Here's how the part is built. I have some questions about the finished solid (model axes, mm). A direction names the side the tool comes from. Give positions to 0.01 mm unless a question says otherwise; leave off trailing zeros. Loops run counter-clockwise (first coordinate to the right, second up) from the corner with the lowest first, then second, coordinate; pieces in that order, holes last. Notation, with made-up numbers: (43.25, 23) - (61.25, 23) arc R15 cw to (61.25, 51) - close; hole circle Ø2 at (-15.75, 38.25). An arc over 180 degrees is marked (long way). Use one line per item in the form item = value.
from build123d import *
from build123d.topology import SkipClean

# Parameters (mm, degrees)
ESBO_O1_R                = 11.15
RESSALTO_EXTRUS_O1_DEPTH = 15
ESBO_O2_R                = 22.5
RESSALTO_EXTRUS_O2_DEPTH = 4
RESSALTO_EXTRUS_O6_START = -8
ESBO_O5_R                = 11.15
ESBO_O5_R_2              = 8
RESSALTO_EXTRUS_O6_DEPTH = 8
RESSALTO_EXTRUS_O7_START = 4
ESBO_O7_R                = 14.2
ESBO_O7_R_2              = 11.15
RESSALTO_EXTRUS_O7_DEPTH = 4
RESSALTO_EXTRUS_O8_START = 4
ESBO_O8_R                = 11.15
ESBO_O8_R_2              = 8
RESSALTO_EXTRUS_O8_DEPTH = 4
RESSALTO_EXTRUS_O9_DEPTH = 7


with BuildPart() as part:
    # Esbo_o1 → Ressalto-extrus_o1 (new body)
    with BuildSketch(Plane.XY):
        with BuildLine():
            Line((-2.5, 18), (-2.5, 13.978197309))
            ThreePointArc((-2.5, 13.978197309), (-10.040916293, 10.040916293), (-13.978197309, 2.5))
            Line((-13.978197309, 2.5), (-18, 2.5))
            Line((-18, 2.5), (-18, -2.5))
            Line((-18, -2.5), (-13.978197309, -2.5))
            ThreePointArc((-13.978197309, -2.5), (-10.040916293, -10.040916293), (-2.5, -13.978197309))
            Line((-2.5, -13.978197309), (-2.5, -18))
            Line((-2.5, -18), (2.5, -18))
            Line((2.5, -18), (2.5, -13.978197309))
            ThreePointArc((2.5, -13.978197309), (10.040916293, -10.040916293), (13.978197309, -2.5))
            Line((13.978197309, -2.5), (18, -2.5))
            Line((18, -2.5), (18, 2.5))
            Line((18, 2.5), (13.978197309, 2.5))
            ThreePointArc((13.978197309, 2.5), (10.040916293, 10.040916293), (2.5, 13.978197309))
            Line((2.5, 13.978197309), (2.5, 18))
            Line((2.5, 18), (-2.5, 18))
        make_face()
        Circle(ESBO_O1_R, mode=Mode.SUBTRACT)
    extrude(amount=RESSALTO_EXTRUS_O1_DEPTH)

    # Esbo_o5 → Ressalto-extrus_o6 (add)
    with BuildSketch(Plane.XY.offset(15).offset(RESSALTO_EXTRUS_O6_START)):
        Circle(ESBO_O5_R)
        Circle(ESBO_O5_R_2, mode=Mode.SUBTRACT)
    extrude(amount=RESSALTO_EXTRUS_O6_DEPTH)



with BuildPart() as body_2:
    # Esbo_o2 → Ressalto-extrus_o2 (new body)
    # profile 1 of 5: a face of its own
    with SkipClean():  # the faces are left unmerged after this step: merging them gives an invalid solid
        with BuildSketch(Plane(origin=(0, 0, 0), x_dir=(-1, 0, 0), z_dir=(0, 0, -1))):
            Circle(ESBO_O2_R)
            with BuildLine():
                Line((2.5, 13.978197309), (2.5, 18))
                Line((2.5, 18), (-2.5, 18))
                Line((-2.5, 18), (-2.5, 13.978197309))
                ThreePointArc((-2.5, 13.978197309), (-10.040916293, 10.040916293), (-13.978197309, 2.5))
                Line((-13.978197309, 2.5), (-18, 2.5))
                Line((-18, 2.5), (-18, -2.5))
                Line((-18, -2.5), (-13.978197309, -2.5))
                ThreePointArc((-13.978197309, -2.5), (-10.040916293, -10.040916293), (-2.5, -13.978197309))
                Line((-2.5, -13.978197309), (-2.5, -18))
                Line((-2.5, -18), (2.5, -18))
                Line((2.5, -18), (2.5, -13.978197309))
                ThreePointArc((2.5, -13.978197309), (10.040916293, -10.040916293), (13.978197309, -2.5))
                Line((13.978197309, -2.5), (18, -2.5))
                Line((18, -2.5), (18, 2.5))
                Line((18, 2.5), (13.978197309, 2.5))
                ThreePointArc((13.978197309, 2.5), (10.040916293, 10.040916293), (2.5, 13.978197309))
            make_face(mode=Mode.SUBTRACT)
        # profile 2 of 5: a face of its own
        with BuildSketch(Plane(origin=(0, 0, 0), x_dir=(-1, 0, 0), z_dir=(0, 0, -1))):
            with BuildLine():
                Line((2.5, -18), (2.5, -13.978197309))
                ThreePointArc((2.5, -13.978197309), (0, -14.2), (-2.5, -13.978197309))
                Line((-2.5, -13.978197309), (-2.5, -18))
                Line((-2.5, -18), (2.5, -18))
            make_face()
        # profile 3 of 5: a face of its own
        with BuildSketch(Plane(origin=(0, 0, 0), x_dir=(-1, 0, 0), z_dir=(0, 0, -1))):
            with BuildLine():
                ThreePointArc((-13.978197309, -2.5), (-14.2, 0), (-13.978197309, 2.5))
                Line((-13.978197309, 2.5), (-18, 2.5))
                Line((-18, 2.5), (-18, -2.5))
                Line((-18, -2.5), (-13.978197309, -2.5))
            make_face()
        # profile 4 of 5: a face of its own
        with BuildSketch(Plane(origin=(0, 0, 0), x_dir=(-1, 0, 0), z_dir=(0, 0, -1))):
            with BuildLine():
                ThreePointArc((-2.5, 13.978197309), (0, 14.2), (2.5, 13.978197309))
                Line((2.5, 13.978197309), (2.5, 18))
                Line((2.5, 18), (-2.5, 18))
                Line((-2.5, 18), (-2.5, 13.978197309))
            make_face()
        # profile 5 of 5: a face of its own
        with BuildSketch(Plane(origin=(0, 0, 0), x_dir=(-1, 0, 0), z_dir=(0, 0, -1))):
            with BuildLine():
                Line((18, 2.5), (13.978197309, 2.5))
                ThreePointArc((13.978197309, 2.5), (14.2, 0), (13.978197309, -2.5))
                Line((13.978197309, -2.5), (18, -2.5))
                Line((18, -2.5), (18, 2.5))
            make_face()
        extrude(amount=RESSALTO_EXTRUS_O2_DEPTH)


with BuildPart() as part_1:
    with SkipClean():  # the faces are left unmerged after this step: merging them gives an invalid solid
        add(part.part)

        add(body_2.part)  # Ressalto-extrus_o7 merges body 2
        # Esbo_o7 → Ressalto-extrus_o7 (add)
        with BuildSketch(Plane(origin=(0, 0, 0), x_dir=(-1, 0, 0), z_dir=(0, 0, -1)).offset(RESSALTO_EXTRUS_O7_START)):
            Circle(ESBO_O7_R)
            with Locations(Location((0, 0, 0), (0, 0, 180))):
                Circle(ESBO_O7_R_2, mode=Mode.SUBTRACT)
        extrude(amount=-RESSALTO_EXTRUS_O7_DEPTH)

    # Esbo_o8 → Ressalto-extrus_o8 (add)
    with BuildSketch(Plane(origin=(0, 0, 7), x_dir=(-1, 0, 0), z_dir=(0, 0, -1)).offset(RESSALTO_EXTRUS_O8_START)):
        Circle(ESBO_O8_R)
        with Locations(Location((0, 0, 0), (0, 0, 180))):
            Circle(ESBO_O8_R_2, mode=Mode.SUBTRACT)
    extrude(amount=-RESSALTO_EXTRUS_O8_DEPTH)

    # Esbo_o9 → Ressalto-extrus_o9 (add)
    with BuildSketch(Plane.XY.offset(15)):
        with BuildLine():
            Line((-11.419478117, 5.324990098), (-8.609923977, 4.014873487))
            ThreePointArc((-8.609923977, 4.014873487), (0, 9.5), (8.609923977, 4.014873487))
            Line((8.609923977, 4.014873487), (11.419478117, 5.324990098))
            ThreePointArc((11.419478117, 5.324990098), (0, 12.6), (-11.419478117, 5.324990098))
        make_face()
        with BuildLine():
            Line((-11.419478117, -5.324990098), (-8.609923977, -4.014873487))
            ThreePointArc((-8.609923977, -4.014873487), (0, -9.5), (8.609923977, -4.014873487))
            Line((8.609923977, -4.014873487), (11.419478117, -5.324990098))
            ThreePointArc((11.419478117, -5.324990098), (0, -12.6), (-11.419478117, -5.324990098))
        make_face()
    extrude(amount=RESSALTO_EXTRUS_O9_DEPTH)


solid = part_1.part
(1) If we section it at B-B (z = 2): List the corners of the cut face in (x, y) for me, plus the area to 3 significant figures.
Geometry says:
outline = (-18, -2.5) - (-13.98, -2.5) arc R14.2 ccw to (-2.5, -13.98) - (-2.5, -18) - (2.5, -18) - (2.5, -13.98) arc R14.2 ccw to (13.98, -2.5) - (18, -2.5) - (18, 2.5) - (13.98, 2.5) arc R14.2 ccw to (2.5, 13.98) - (2.5, 18) - (-2.5, 18) - (-2.5, 13.98) arc R14.2 ccw to (-13.98, 2.5) - (-18, 2.5) - close; hole circle Ø22.3 at (0, 0)
area = 320 mm²
(2) For faces 4 (the flat face through (-10.034, 4.679, 18.451)), 5 (the flat face through (9.995, -4.661, 18.451)), 6 (the flat face through (-5, -15, 0)), 7 (the cylindrical face through (-9.955, 10.126, 7.395)), 8 (the flat face through (-18, 0, 7)), which set-ups out of +Z, -Z, +X, -X, +Y, -Y let a thin tool reach every point of the face, with its end or its side?
Geometry says:
face_4 = +Z, -X
face_5 = +Z, +X
face_6 = +Z
face_7 = +Z, -X, +Y
face_8 = +Z, -X, +Y, -Y
(3) If we section it at C-C (x = 0): List the corners of the cut face in (y, z) for me.
Geometry says:
outline = (-22.5, -4) - (-11.15, -4) - (-11.15, 3) - (-8, 3) - (-8, 15) - (-9.5, 15) - (-9.5, 22) - (-12.6, 22) - (-12.6, 15) - (-18, 15) - (-18, 0) - (-22.5, 0) - close; (8, 3) - (11.15, 3) - (11.15, -4) - (22.5, -4) - (22.5, 0) - (18, 0) - (18, 15) - (12.6, 15) - (12.6, 22) - (9.5, 22) - (9.5, 15) - (8, 15) - close
(4) Thinking about a two-plate mould opening in Y: for faces 1 (the cylindrical face through (-0.15, 9.5, 18.45)), 2 (the flat face through (0, 10, 22)), 3 (the cylindrical face through (9.955, -10.126, 7.395)), which applies, pulls with the +Y half, pulls with the -Y half, needs draft (parallel to the pull), parting line crosses it, or undercut?
Geometry says:
face_1 = undercut
face_2 = needs draft
face_3 = pulls with the -Y half
(5) If we section it at A-A (y = 0): List the corners of the cut face in (x, z) for me, plus the area to 3 significant figures.
Geometry says:
outline = (-22.5, -4) - (-11.15, -4) - (-11.15, 3) - (-8, 3) - (-8, 15) - (-18, 15) - (-18, 0) - (-22.5, 0) - close; (8, 3) - (11.15, 3) - (11.15, -4) - (22.5, -4) - (22.5, 0) - (18, 0) - (18, 15) - (8, 15) - close
area = 372 mm²
(6) If I drill on probe 1 along Y at (x, z) = (0, 4.7); probe 2 along Y at (x, z) = (0, -2.55); probe 3 along Z at (x, y) = (-11, -12.5), over which ranges is the centre line in solid material (lowest first)?
Geometry says:
probe_1 = -18 to -8, 8 to 18
probe_2 = -22.5 to -11.15, 11.15 to 22.5
probe_3 = -4 to 0
(7) For P1, Ø1.2, axis at y = 16, z = 8, coming from the +X side; P2, Ø18.5, axis at x = 0, y = 0, coming from the +Z side; P3, Ø18, axis at x = 0, y = 0, coming from the -Z side; P4, Ø13, axis at x = 0, y = 0, coming from the +Z side, each with a flat end and sliding along its axis, tell me the tip position at first contact or that it passes through.
Geometry says:
P1 = 2.5
P2 = 15
P3 = 3
P4 = through
(8) If we section it at D-D (z = 5.5): List the corners of the cut face in (x, y) for me, plus the area to 3 significant figures.
Geometry says:
outline = (-18, -2.5) - (-13.98, -2.5) arc R14.2 ccw to (-2.5, -13.98) - (-2.5, -18) - (2.5, -18) - (2.5, -13.98) arc R14.2 ccw to (13.98, -2.5) - (18, -2.5) - (18, 2.5) - (13.98, 2.5) arc R14.2 ccw to (2.5, 13.98) - (2.5, 18) - (-2.5, 18) - (-2.5, 13.98) arc R14.2 ccw to (-13.98, 2.5) - (-18, 2.5) - close; hole circle Ø16 at (0, 0)
area = 510 mm²
